Here's how the part is built. I have some questions about the finished solid (model axes, mm). A direction names the side the tool comes from. Coordinates: 2 decimals unless noted, no trailing zeros. Write each loop counter-clockwise with the first axis right and the second up, starting at its lowest first coordinate (ties: lowest second). Pieces come first, ordered by that corner, then holes. Notation, with made-up numbers: M 0.5,58 L 54.5,58 A18 ccw 54.5,88 Z; hole C 2,61.25 d11. An arc over 180 degrees is marked long. Use a Markdown table: item, result.
```python
from build123d import *

# Parameters (mm, degrees)
SKETCH1_R           = 1.75
SKETCH1_W           = 16
SKETCH1_H           = 5.5
BOSS_EXTRUDE1_DEPTH = 3


with BuildPart() as part:
    # Sketch1 → Boss-Extrude1 (new body)
    with BuildSketch(Plane.XY):
        with BuildLine():
            Line((-3.6, 18.5), (3.6, 18.5))
            ThreePointArc((3.6, 18.5), (5.721320344, 17.621320344), (6.6, 15.5))
            Line((6.6, 15.5), (6.6, -15.5))
            Line((6.6, -15.5), (-6.6, -15.5))
            Line((-6.6, -15.5), (-6.6, 15.5))
            ThreePointArc((-6.6, 15.5), (-5.721320344, 17.621320344), (-3.6, 18.5))
        make_face()
        with Locations((0, 12.5)):
            Circle(SKETCH1_R, mode=Mode.SUBTRACT)
        with BuildLine():
            Line((1.75, -3), (1.75, -6))
            ThreePointArc((1.75, -6), (0, -7.75), (-1.75, -6))
            Line((-1.75, -6), (-1.75, -3))
            ThreePointArc((-1.75, -3), (0, -1.25), (1.75, -3))
        make_face(mode=Mode.SUBTRACT)
        with Locations((0, -12.75)):
            Rectangle(SKETCH1_W, SKETCH1_H)
    extrude(amount=BOSS_EXTRUDE1_DEPTH)


solid = part.part
```
1. Will these pins go through, and if not, where does the flat tip stop? pin 1 Ø2 at (x, y) = (0, 12.5) entering from +Z; pin 2 Ø1.5 at (y, z) = (5.5, 1) entering from -X.
Answers follow:
| item | result |
|---|---|
| pin 1 | passes through |
| pin 2 | stops at x = -6.6 |
2. Suppose I cut it at C-C on x = 0. Write out the boundary of the cut face in (y, z), and give its area (3 significant figures).
Answers follow:
| item | result |
|---|---|
| outline | M -15.5,0 L -7.75,0 L -7.75,3 L -15.5,3 Z; M -1.25,0 L 10.75,0 L 10.75,3 L -1.25,3 Z; M 14.25,0 L 18.5,0 L 18.5,3 L 14.25,3 Z |
| area | 72.0 mm2 |
3. Suppose I cut it at A-A on y = 12.5. Write out the boundary of the cut face in (x, z).
Answers follow:
| item | result |
|---|---|
| outline | M -6.6,0 L -1.75,0 L -1.75,3 L -6.6,3 Z; M 1.75,0 L 6.6,0 L 6.6,3 L 1.75,3 Z |
4. Suppose I cut it at D-D on y = -2.5. Write out the boundary of the cut face in (x, z).
Answers follow:
| item | result |
|---|---|
| outline | M -6.6,0 L -1.68,0 L -1.68,3 L -6.6,3 Z; M 1.68,0 L 6.6,0 L 6.6,3 L 1.68,3 Z |
5. We'd pull the mould along Y, two halves only. Please class faces 1 (the face through (5.7, 17.64, 1.48)), 2 (the face through (0, -15.5, 1)), 3 (the face through (-8, -13, 1)), 4 (the face through (-0.228, 14.235, 1.479)): +Y half, -Y half, draft (parallel to the pull), parting line (faces both ways), or undercut.
Answers follow:
| item | result |
|---|---|
| face 1 | +Y half |
| face 2 | -Y half |
| face 3 | draft |
| face 4 | undercut |
6. I need wall thicknesses on probe 1 along Y at (x, z) = (0, 0.7); probe 2 along X at (y, z) = (-5, 1.95); probe 3 along Y at (x, z) = (1, 2.4). Which ranges of each line are inside material? Lowest first, please.
Answers follow:
| item | result |
|---|---|
| probe 1 | y = -15.5 to -7.75, -1.25 to 10.75, 14.25 to 18.5 |
| probe 2 | x = -6.6 to -1.75, 1.75 to 6.6 |
| probe 3 | y = -15.5 to -7.44, -1.56 to 11.06, 13.94 to 18.5 |
7. Suppose I cut it at B-B on z = 1.8. Write out the boundary of the cut face in (x, y).
Answers follow:
| item | result |
|---|---|
| outline | M -8,-15.5 L 8,-15.5 L 8,-10 L 6.6,-10 L 6.6,15.5 A3 ccw 3.6,18.5 L -3.6,18.5 A3 ccw -6.6,15.5 L -6.6,-10 L -8,-10 Z; hole M -1.75,-6 A1.75 ccw 1.75,-6 L 1.75,-3 A1.75 ccw -1.75,-3 Z; hole C 0,12.5 d3.5 |
8. Which directions (+Z, -Z, +X, -X, +Y, -Y) give clear straight access to the entire face, cutting with the end or side of a thin tool? Please do faces 5 (the face through (1.75, -4, 1)), 6 (the face through (-7, -10, 1)), 7 (the face through (8, -13, 1)), 8 (the face through (0, 2, 0)), 9 (the face through (7, -10, 1)).
Answers follow:
| item | result |
|---|---|
| face 5 | +Z, -Z |
| face 6 | +Z, -Z, -X, +Y |
| face 7 | +Z, -Z, +X, +Y, -Y |
| face 8 | -Z, +X, -X, +Y, -Y |
| face 9 | +Z, -Z, +X, +Y |
